from build123d import *

# Parameters (mm, degrees)
F0_R           = 15.1824843522
F0_R_2         = 12
F1_DEPTH       = 20
F0_R_3         = 21.6830909865
F2_DEPTH       = 20
F3_R           = 6.3
F0_R_4         = 27.1312843312
F4_DEPTH       = 14
F5_S5_R        = 21.6830909865
F5_T6_DEPTH    = 40
F0_R_5         = 1.775
F6_DEPTH       = 4
F8_D           = 2.7
F8_DEPTH       = 12
F8_CSINK_D     = 7
F8_CSINK_ANGLE = 66
F8_TIP         = 0.8111618357


# Not quite as in the source:
# - a fillet or chamfer that OpenCascade refuses, or shapes differently, is made with other operations: its cross-section is extruded or revolved along the edge and cut away or added


with BuildPart() as f1:
    # F0 (on Right) → F1 (new body)
    with BuildSketch(Plane.YZ):
        Circle(F0_R)
        Circle(F0_R_2, mode=Mode.SUBTRACT)
    extrude(amount=F1_DEPTH)

    # F0 (on Right) → F2 (join)
    with BuildSketch(Plane.YZ):
        Circle(F0_R_3)
        Circle(F0_R, mode=Mode.SUBTRACT)
    extrude(amount=F2_DEPTH)

    # F3
    f3_edges = [f1.edges().sort_by_distance(p)[0] for p in [
        (20, -21.683091, 0),
    ]]
    fillet(f3_edges, radius=F3_R)

    # F0 (on Right) → F4 (join)
    with BuildSketch(Plane.YZ):
        Circle(F0_R_4)
        Circle(F0_R_3, mode=Mode.SUBTRACT)
    extrude(amount=F4_DEPTH)

    # F5: chamfer of 5.5 x 12.3532022565 on 1 edges, made by hand


with BuildPart() as f5_tool2:
    # F5_s3 → F5_t4 (revolve)
    with BuildSketch(Plane.XY):
        Polygon((14, 21.6312843312), (1.6467977435, 27.1312843312), (14, 27.1312843312), align=None)
    revolve(axis=Axis((14, 0, 0), (1, 0, 0)))

    # F5_s5 → F5_t6 (cut, symmetric)
    with BuildSketch(Plane.YZ.offset(7.8)):
        Circle(F5_S5_R)
    extrude(amount=F5_T6_DEPTH, both=True, mode=Mode.SUBTRACT)


with BuildPart() as f1_1:
    add(f1.part)

    # F5_t1: cut F5_tool2
    add(f5_tool2.part, mode=Mode.SUBTRACT)

    # F0 (on Right) → F6 (join)
    with BuildSketch(Plane.YZ):
        Circle(F0_R_2)
        Circle(F0_R_5, mode=Mode.SUBTRACT)
        Circle(F0_R_5)
    extrude(amount=F6_DEPTH)

    # F8
    with Locations(Plane.YZ.offset(4)):
        with Locations((0, 0)):
            CounterSinkHole(F8_D / 2, F8_CSINK_D / 2, depth=F8_DEPTH, counter_sink_angle=F8_CSINK_ANGLE)
            with Locations((0, 0, -(F8_DEPTH + F8_TIP / 2))):  # 118° drill point
                Cone(0, F8_D / 2, F8_TIP, mode=Mode.SUBTRACT)


solid = f1_1.part
Design review of the part built by this model. Coordinates are the model's own, in mm. A direction names the side the tool comes from. Round coordinates to 2 decimals unless told otherwise and drop trailing zeros. Loops run counter-clockwise (first coordinate to the right, second up) from the corner with the lowest first, then second, coordinate; pieces in that order, holes last. Notation, with made-up numbers: (33, -30.5) -> (46, -30.5) arc R22 ccw to (46, -7.5) -> close; hole circle Ø9 at (10.5, 30). An arc over 180 degrees is marked (long way). Use one line per item in the form item = value. Start each with the question number.
Q1. We need section D-D on x = 3. Give the boundary of the cut face in (y, z).
Q2. For pin 1 Ø1.6 at (y, z) = (0, 0) entering from +X; pin 2 Ø5 at (x, z) = (11, -8) entering from -Y; pin 3 Ø4 at (x, z) = (7, 2.5) entering from +Y; pin 4 Ø2 at (x, z) = (7, -3.5) entering from -Y, all flat-tipped, find the tip position at first contact; note any pin that passes through.
Q3. We need section A-A on y = 0. Give the boundary of the cut face in (x, z).
Q4. We need section C-C on x = 17.25. Give the boundary of the cut face in (y, z), then the cut area to 3 significant figures.
Q5. Draft analysis for pull direction Z (two halves, no side actions). For faces 3 (the face through (20, -4.6, -11.3)), 4 (the face through (0.34, 0.29, -1.32)), 5 (the face through (13.12, -4.77, -21.5)), state which applies: +Z half, -Z half, draft (parallel to the pull), parting line (faces both ways), or undercut.
Q6. Machinability: for faces 1 (the face through (11.89, -11.99, 0.53)), 2 (the face through (0.81, -3.53, 26.9)), which of the approach directions +Z, -Z, +X, -X, +Y, -Y give a long, thin tool a straight path to every point of the face, cutting with its end or side? Answer none if there is none.
Q7. Wall thickness on line 1 along X through (y, z) = (-10, -4.5); line 2 along Z through (x, y) = (16.25, -2); line 3 along Z through (x, y) = (0.2, 0): over which ranges is each line inside the solid? List them lowest first. Write a range as [from, to].
Calculated:
q1.outline = circle Ø53.06 at (0, 0); hole circle Ø5.7 at (0, 0)
q2.pin_1 = through
q2.pin_2 = -22.96
q2.pin_3 = 25.53
q2.pin_4 = -24.97
q3.outline = (0, -27.13) -> (1.65, -27.13) -> (13.88, -21.68) -> (13.7, -21.68) arc R6.3 ccw to (20, -15.38) -> (20, -12) -> (4, -12) -> (4, -3.5) -> (0.69, -1.35) -> (0, -1.35) -> close; (0, 1.35) -> (0.69, 1.35) -> (4, 3.5) -> (4, 12) -> (20, 12) -> (20, 15.38) arc R6.3 ccw to (13.7, 21.68) -> (13.88, 21.68) -> (1.65, 27.13) -> (0, 27.13) -> close
q4.outline = circle Ø41.18 at (0, 0); hole circle Ø24 at (0, 0)
q4.area = 879 mm²
q5.face_3 = draft
q5.face_4 = undercut
q5.face_5 = parting line
q6.face_1 = +X
q6.face_2 = +X, -X
q7.line_1 = [0, 4]
q7.line_2 = [-21.05, -11.83], [11.83, 21.05]
q7.line_3 = [-27.13, -1.35], [1.35, 27.13]
